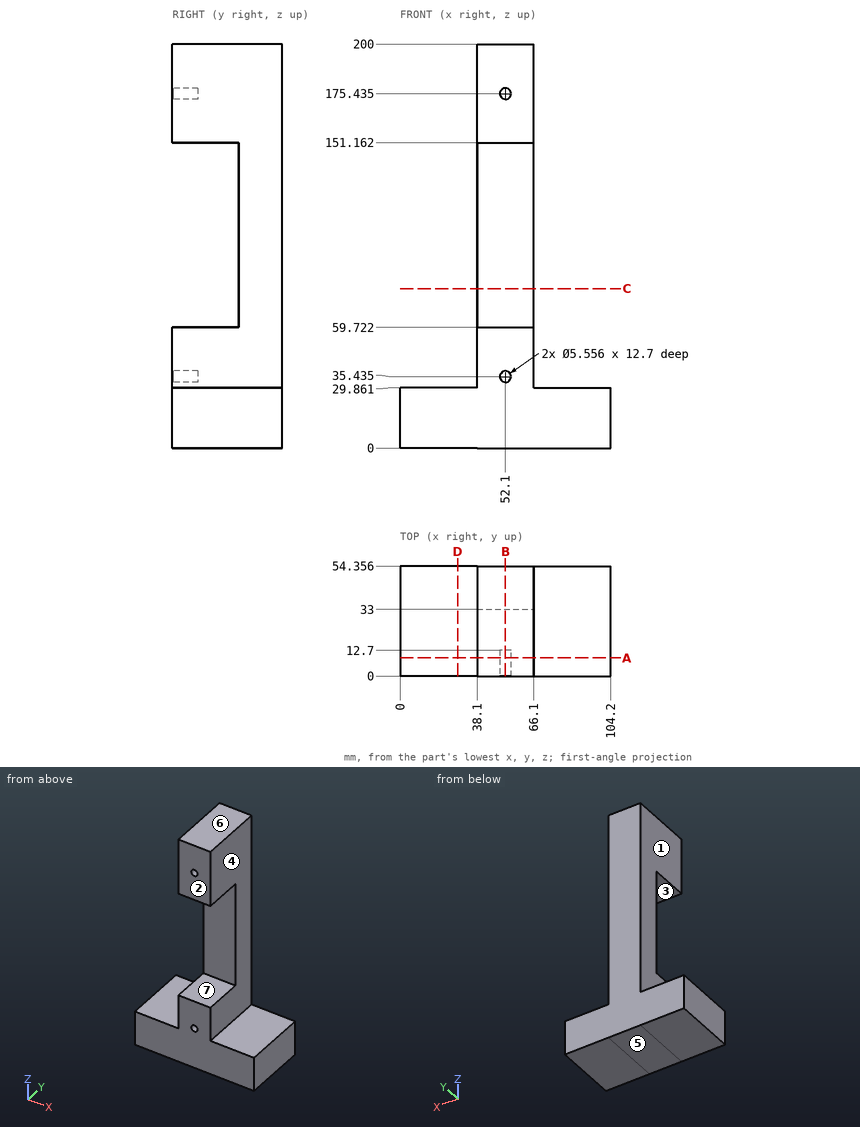
Answer from the drawing. Dimensions are ordinates in mm from the lowest x, y and z of the part. A direction names the side the tool comes from. Give positions to 0.01 mm unless a question says otherwise; leave off trailing zeros. Loops run counter-clockwise (first coordinate to the right, second up) from the corner with the lowest first, then second, coordinate; pieces in that order, holes last. Notation, with made-up numbers: (37, -35) - (54, -35) arc R22 ccw to (54, -23) - close; hole circle Ø9 at (34, -14). An arc over 180 degrees is marked (long way). Answer as CSV lines item,"result". Start each with the question number.
Item 1: For the marked faces 1, 2, 3 and 4, determine the directions among +Z, -Z, +X, -X, +Y, -Y from which every point of the face is accessible in a straight line to the end or side of a thin tool.
Item 2: A cutting plane is placed at A-A on y = 9. Determine the outline of the cut face in (x, z) (1 decimal).
Item 3: A cutting plane is placed at D-D on x = 28.5. Determine the outline of the cut face in (y, z), then the cut area to 3 significant figures.
Item 4: The mould has two halves that part along Z. Classify the marked faces 5, 6 and 7: +Z half, -Z half, draft (parallel to the pull), parting line (faces both ways), or undercut.
Item 5: Each of these flat-tipped pins is pushed along its axis until it touches: pin 1 (1.7 mm diameter, centred on x = 51.5, z = 34, fed in from -Y); pin 2 (11.5 mm diameter, centred on x = 20.5, y = 34.5, fed in from +Z); pin 3 (2 mm diameter, centred on y = 36, z = 151, fed in from +X). Where does it stop, or does it pass through?
Item 6: A cutting plane is placed at B-B on x = 52.1. Determine the outline of the cut face in (y, z), then the cut area to 3 significant figures.
Item 7: A cutting plane is placed at C-C on z = 79. Determine the outline of the cut face in (x, y), then the cut area to 3 significant figures.
Item 8: Find the intervals of material crossed by line 1 (Z direction, x = 52, y = 5); line 2 (Z direction, x = 56.5, y = 13); line 3 (Z direction, x = 87, y = 31.5), in increasing order. Write a range as from..to.
Found:
1,face 1,"+Z, -X, +Y, -Y"
1,face 2,"+Z, -Z, +X, -X, -Y"
1,face 3,"+X, -X, -Y"
1,face 4,"+Z, +X, +Y, -Y"
2,outline,"(0, 0) - (104.2, 0) - (104.2, 29.9) - (66.1, 29.9) - (66.1, 59.7) - (38.1, 59.7) - (38.1, 29.9) - (0, 29.9) - close; (38.1, 151.2) - (66.1, 151.2) - (66.1, 200) - (38.1, 200) - close; hole circle Ø5.6 at (52.1, 35.4); hole circle Ø5.6 at (52.1, 175.4)"
3,outline,"(0, 0) - (54.36, 0) - (54.36, 29.86) - (0, 29.86) - close"
3,area,"1,620 mm^2"
4,face 5,"-Z half"
4,face 6,"+Z half"
4,face 7,"undercut"
5,pin 1,"stops at y = 12.7"
5,pin 2,"stops at z = 29.86"
5,pin 3,"stops at x = 66.1"
6,outline,"(0, 0) - (54.36, 0) - (54.36, 200) - (0, 200) - (0, 178.21) - (12.7, 178.21) - (12.7, 172.66) - (0, 172.66) - (0, 151.16) - (33, 151.16) - (33, 59.72) - (0, 59.72) - (0, 38.21) - (12.7, 38.21) - (12.7, 32.66) - (0, 32.66) - close"
6,area,"7,710 mm^2"
7,outline,"(38.1, 33) - (66.1, 33) - (66.1, 54.36) - (38.1, 54.36) - close"
7,area,"598 mm^2"
8,line 1,"z = 0..32.66, 38.21..59.72, 151.16..172.66, 178.21..200"
8,line 2,"z = 0..59.72, 151.16..200"
8,line 3,"z = 0..29.86"
